```python
from build123d import *

# Parameters (mm, degrees)
SKETCH1_W           = 49.276
SKETCH1_H           = 12.192
BOSS_EXTRUDE1_DEPTH = 2
SKETCH2_W           = 53.276
SKETCH2_H           = 16.192
SKETCH2_W_2         = 49.276
SKETCH2_H_2         = 12.192
BOSS_EXTRUDE2_DEPTH = 7
SKETCH3_R           = 2.12725
CUT_EXTRUDE1_DEPTH  = 3
SKETCH5_W           = 25
SKETCH5_H           = 3.25
CUT_EXTRUDE2_DEPTH  = 0.6


with BuildPart() as part:
    # Sketch1 → Boss-Extrude1 (new body)
    with BuildSketch(Plane(origin=(0, 0, 0), x_dir=(1, 0, 0), z_dir=(0, 1, 0))):
        Rectangle(SKETCH1_W, SKETCH1_H)
    extrude(amount=BOSS_EXTRUDE1_DEPTH)

    # Sketch2 → Boss-Extrude2 (add)
    with BuildSketch(Plane(origin=(0, 0, 0), x_dir=(1, 0, 0), z_dir=(0, 1, 0))):
        Rectangle(SKETCH2_W, SKETCH2_H)
        Rectangle(SKETCH2_W_2, SKETCH2_H_2, mode=Mode.SUBTRACT)
    extrude(amount=BOSS_EXTRUDE2_DEPTH)

    # Sketch3 → Cut-Extrude1 (cut, through all)
    with BuildSketch(Plane(origin=(0, 2, 0), x_dir=(1, 0, 0), z_dir=(0, 1, 0))):
        with Locations((-18.542, 0)):
            Circle(SKETCH3_R)
    cut_extrude1 = extrude(amount=-CUT_EXTRUDE1_DEPTH, mode=Mode.SUBTRACT)

    # Sketch4 → Cut-Revolve1 (revolve, cut)
    with BuildSketch(Plane(origin=(0, 0, 0), x_dir=(-1, 0, 0), z_dir=(0, 0, -1))):
        Polygon((18.542, 1), (18.542, 2), (14.57325, 2), (18.542, -1.96875), align=None)
    cut_revolve1 = revolve(axis=Axis((-18.542, 2, 0), (0, 1, 0)), mode=Mode.SUBTRACT)

    # Mirror1: Cut-Extrude1, Cut-Revolve1 across plane
    add(cut_extrude1.mirror(Plane(origin=(0, 0, 0), x_dir=(0, 0, 1), z_dir=(1, 0, 0))), mode=Mode.SUBTRACT)
    add(cut_revolve1.mirror(Plane(origin=(0, 0, 0), x_dir=(0, 0, 1), z_dir=(1, 0, 0))), mode=Mode.SUBTRACT)

    # Sketch5 → Cut-Extrude2 (cut)
    with BuildSketch(Plane(origin=(0, 0, 0), x_dir=(-1, 0, 0), z_dir=(0, -1, 0))):
        with Locations((0, -5.471)):
            Rectangle(SKETCH5_W, SKETCH5_H)
        with Locations((0, 5.471)):
            Rectangle(SKETCH5_W, SKETCH5_H)
    extrude(amount=-CUT_EXTRUDE2_DEPTH, mode=Mode.SUBTRACT)


solid = part.part
```
Work out the finished part from the listing and answer in its coordinate system (mm). A direction names the side the tool comes from. Round coordinates to 2 decimals unless told otherwise and drop trailing zeros. Write each loop counter-clockwise with the first axis right and the second up, starting at its lowest first coordinate (ties: lowest second). Pieces come first, ordered by that corner, then holes. Notation, with made-up numbers: (63.25, 8) -> (68.25, 8) arc R8 ccw to (68.25, 16) -> close; hole circle Ø5 at (-26.75, 72). An arc over 180 degrees is marked (long way). Write each question's results on one line, items separated by ' | '.
1) For a pull along X with two mould halves and no side action, classify faces 1 (the flat face through (0, 3, -8.096)), 2 (the flat face through (-26.638, 3, 0)), 3 (the flat face through (0, 0.6, 5)) as +X half, -X half, draft (parallel to the pull), parting line (faces both ways), or undercut.
Findings:
face 1: draft | face 2: -X half | face 3: undercut
2) The part is cut by section C-C (z = -5). Write down the section's boundary in (x, y), and give its area (3 significant figures).
Findings:
outline: (-26.64, 0) -> (-12.5, 0) -> (-12.5, 0.6) -> (12.5, 0.6) -> (12.5, 0) -> (26.64, 0) -> (26.64, 7) -> (24.64, 7) -> (24.64, 2) -> (-24.64, 2) -> (-24.64, 7) -> (-26.64, 7) -> close | area: 112 mm²
3) The part is cut by section A-A (z = 0). Write down the section's boundary in (x, y).
Findings:
outline: (-26.64, 0) -> (-20.67, 0) -> (-20.67, 0.16) -> (-22.51, 2) -> (-24.64, 2) -> (-24.64, 7) -> (-26.64, 7) -> close; (-16.41, 0) -> (16.41, 0) -> (16.41, 0.16) -> (14.57, 2) -> (-14.57, 2) -> (-16.41, 0.16) -> close; (20.67, 0) -> (26.64, 0) -> (26.64, 7) -> (24.64, 7) -> (24.64, 2) -> (22.51, 2) -> (20.67, 0.16) -> close
4) The part is cut by section B-B (y = 2.5). Write down the section's boundary in (x, z), and give its area (3 significant figures).
Findings:
outline: (-26.64, -8.1) -> (26.64, -8.1) -> (26.64, 8.1) -> (-26.64, 8.1) -> close; hole (-24.64, -6.1) -> (24.64, -6.1) -> (24.64, 6.1) -> (-24.64, 6.1) -> close | area: 262 mm²
5) A flat-ended cylindrical pin translates along its axis: pin 1 (3 mm diameter, centred on x = 5, z = -5.5, fed in from -Y). Find the tip coordinate at first contact, or state that the pin passes through.
Findings:
pin 1: stops at y = 0.6
6) Consider line 1 along Z through (x, y) = (7, 0.5); line 2 along Z through (x, y) = (16, 2.5); line 3 along X through (y, z) = (3, -2.5). Determine where each line is inside the solid, lowest interval first. Write a range as [from, to].
Findings:
line 1: z = [-8.1, -7.1], [-3.85, 3.85], [7.1, 8.1] | line 2: z = [-8.1, -6.1], [6.1, 8.1] | line 3: x = [-26.64, -24.64], [24.64, 26.64]
7) Which of the six approach directions +Z, -Z, +X, -X, +Y, -Y give full straight-line access (tool end or side, diameter ignored) to faces 4 (the flat face through (0, 0.6, -5)), 5 (the flat face through (0, 3, 8.096)), 6 (the flat face through (24.638, 4, 0))?
Findings:
face 4: -Y | face 5: +Z, +X, -X, +Y, -Y | face 6: +Y
8) The part is cut by section D-D (x = -6.5). Write down the section's boundary in (y, z), and give its area (3 significant figures).
Findings:
outline: (0, -8.1) -> (7, -8.1) -> (7, -6.1) -> (2, -6.1) -> (2, 6.1) -> (7, 6.1) -> (7, 8.1) -> (0, 8.1) -> (0, 7.1) -> (0.6, 7.1) -> (0.6, 3.85) -> (0, 3.85) -> (0, -3.85) -> (0.6, -3.85) -> (0.6, -7.1) -> (0, -7.1) -> close | area: 48.5 mm²
